Could you check a few things on this drawing? It's one solid part, dimensions in mm from its lowest x, y, z. A direction names the side the tool comes from. Give positions to 0.01 mm unless a question says otherwise; leave off trailing zeros. Order: outer loops, then holes, each group sorted by start corner. A loop starts at its lowest first (then second) coordinate and runs counter-clockwise, first axis right, second up.
(1) Imagine slicing it at B-B, the plane z = 7.5. Write out the boundary of the cut face in (x, y), then the cut area to 3 significant figures.
(2) Will these pins go through, and if not, where does the flat tip stop? pin 1 (10 mm diameter, centred on x = 21, z = 14, fed in from -Y); pin 2 (9.5 mm diameter, centred on x = 25, y = 25, fed in from -Z).
(3) If we mould it in two halves opening along X, with no side actions, what happens to the marked faces 1, 2, 3 and 4? For each: released by +X, released by -X, zero draft, split by the parting line, or undercut.
(4) On a 3-axis mill with a long thin cutter (end or side, diameter ignored), from which of +Z, -Z, +X, -X, +Y, -Y can I reach the whole of each face in a straight line? I mean the marked faces 5, 6 and 7. Say none if no direction works.
(5) Imagine slicing it at A-A, the plane x = 35.5. Write out the boundary of the cut face in (y, z), then the cut area to 3 significant figures.
(6) If I drill on probe 1 along X at (y, z) = (25, 2.35); probe 2 along Z at (x, y) = (42, 10.5) (1 decimal); probe 3 along Y at (x, z) = (25, 3.1), over which ranges is the centre line in solid material (lowest first)?
(7) Imagine slicing it at C-C, the plane z = 1.5. Write out the boundary of the cut face in (x, y), then the cut area to 3 significant figures.
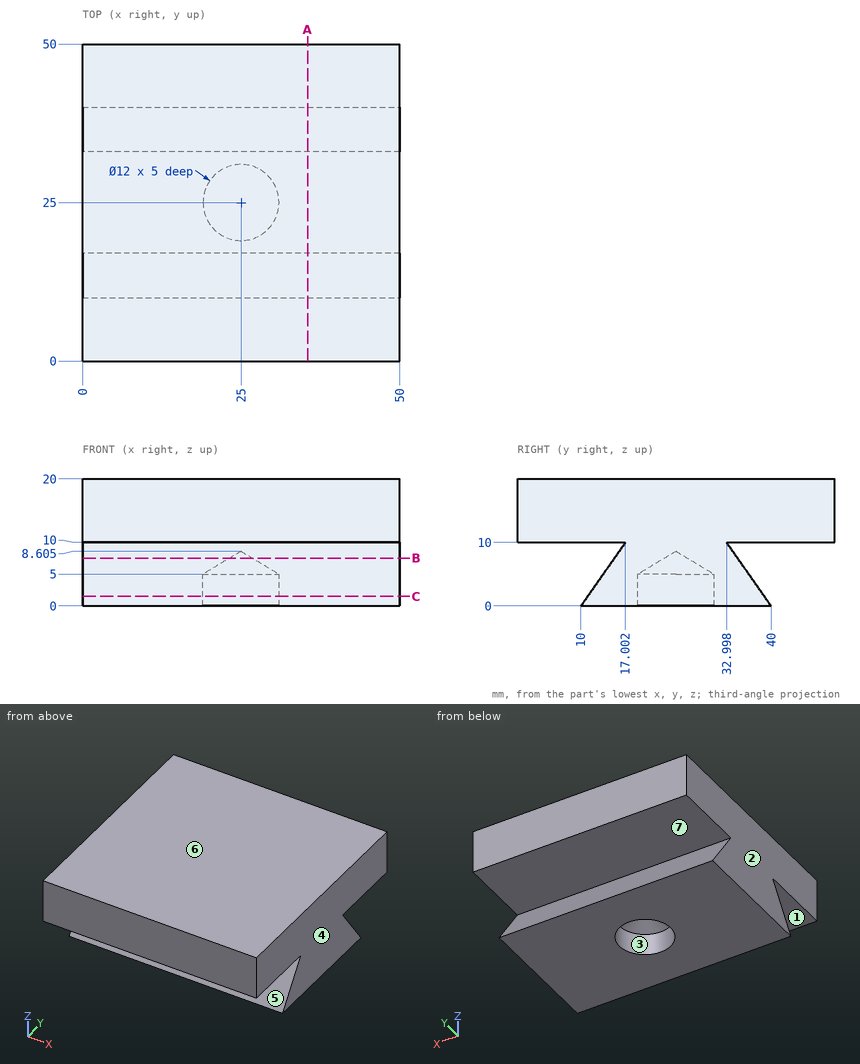
Answer block:
1. outline: (0, 15.25) - (50, 15.25) - (50, 34.75) - (0, 34.75) - close; hole circle Ø3.68 at (25, 25)
1. area: 964 mm2
2. pin 1: stops at y = 0
2. pin 2: stops at z = 5.75
3. face 1: zero draft
3. face 2: released by -X
3. face 3: undercut
3. face 4: released by +X
4. face 5: +X, -X, -Y
4. face 6: +Z, +X, -X, +Y, -Y
4. face 7: +X, -X, +Y
5. outline: (0, 10) - (17, 10) - (10, 0) - (40, 0) - (33, 10) - (50, 10) - (50, 20) - (0, 20) - close
5. area: 730 mm2
6. probe 1: x = 0 to 19, 31 to 50
6. probe 2: z = 0 to 0.7, 10 to 20
6. probe 3: y = 12.17 to 19, 31 to 37.83
7. outline: (0, 11.05) - (50, 11.05) - (50, 38.95) - (0, 38.95) - close; hole circle Ø12 at (25, 25)
7. area: 1,280 mm2
